Build history of the part. All positions in model axes, mm. Face numbers are marked on the shaded views. A direction names the side the tool comes from. Coordinates: 2 decimals unless noted, no trailing zeros. Loops run counter-clockwise (first coordinate to the right, second up) from the corner with the lowest first, then second, coordinate; pieces in that order, holes last.
Item 1: 3-axis set-ups, long thin cutter, end or side, ignore diameter. For the marked faces 1 and 2: which of +Z, -Z, +X, -X, +Y, -Y reach the whole face in a straight line?
Item 2: Cut at B-B (x = 44.5). List the corners of the cut face in (y, z) (1 decimal).
Item 3: Cut at A-A (x = -2.5). List the corners of the cut face in (y, z), and give its area (3 significant figures).
Item 4: Flat gauge pins, fed straight in: pin 1 (12 mm diameter, centred on x = 22.5, y = 11.5, fed in from -Z); pin 2 (2 mm diameter, centred on x = 75, z = -10, fed in from -Y); pin 3 (5 mm diameter, centred on y = 11, z = -5.5, fed in from +X). Where does each tip first touch, or does it go through?
Item 5: Drill centre lines: line 1 along X through (y, z) = (11.5, -8); line 2 along Z through (x, y) = (53, 0); line 3 along Y through (x, z) = (8, 3.5). Where is each one in solid material? Low to high.
Autodesk Inventor part; units mm, degrees
ref_plane "Work Plane1" through (1.525, 0, 0) normal (0, 0, 1) x (1, 0, 0)
ref_plane "YZ Plane" through (0, 0, 0) normal (1, 0, 0) x (0, 1, 0)
ref_plane "XZ Plane" through (0, 0, 0) normal (0, 1, 0) x (-1, 0, 0)
sketch "Sketch1" plane through (0, 0, 0) normal (0, 0, 1) x (1, 0, 0)
  line L0 (0, 16.4306) -> (0, 11.1125)
  line L1 (63.5, 11.1125) -> (101.6, 11.1125)
  line L2 (101.6, 11.1125) -> (101.6, 0)
  line L3 (101.6, 0) -> (-0.6351, 0)
  line L4 (-21.0821, 0) -> (122.047, 0)
  line L5 (-0.6351, 0) -> (-0.6351, 16.4306)
  line L6 (-0.6351, 16.4306) -> (0, 16.4306)
  line L7 (63.5, 11.1125) -> (61.7685, 11.1125)
  line L8 (61.7685, 11.1125) -> (0, 11.1125)
  line L9 (0, -3.2861) -> (0, 19.7168)
  dimension "d0" = 101.6
  dimension "d1" = 38.1
  dimension "d2" = 22.225
  dimension "d9" = 0.6351
  dimension "d10" = 32.8612
  dimension "d13" = 1.7315
  dimension "d14" = 22.225
revolve "Body" add sketch "Sketch1" angle 360 about axis through (101.6, 0, 0) along (-1, 0, 0)
sketch "Sketch2" plane through (-0.6351, 0, 0) normal (-1, 0, 0) x (0, 0, 1)
  line L0 (0, 21.0805) -> (18.2562, 10.5403)
  line L1 (18.2562, 10.5403) -> (18.2562, -10.5403)
  line L2 (18.2562, -10.5403) -> (0, -21.0805)
  line L3 (0, -21.0805) -> (-18.2562, -10.5403)
  line L4 (-18.2562, -10.5403) -> (-18.2562, 10.5403)
  line L5 (-18.2562, 10.5403) -> (0, 21.0805)
  point P0 (0, 0)
  point P1 (0, 0)
  dimension "d11" = 36.5125
extrude "Head" add sketch "Sketch2" along normal blind 13.2556
sketch "Sketch4" plane through (0, 0, 0) normal (0, 0, 1) x (1, 0, 0)
  line L0 (-13.8907, 18.2563) -> (-13.8907, 21.0805)
  line L1 (-13.8907, 21.0805) -> (-12.2601, 21.0805)
  line L2 (-12.2601, 21.0805) -> (-13.8907, 18.2563)
  line L3 (-16.5419, 0) -> (2.016, 0)
  line L4 (-0.6351, 21.0805) -> (-13.8907, 21.0805)
  line L5 (-13.8907, 10.5403) -> (-13.8907, 21.0805)
  dimension "d5" = 30
  dimension "d19" = 36.5125
revolve "Chamfer1" cut sketch "Sketch4" angle 360 about axis through (-10, 0, 0) along (1, 0, 0)
thread "Thread"
chamfer "Chamfer2" distance 1.7314 distance2 1.7315 1 edges at (101.6, -11.1125, 0) measured on face at (101.6, -3.0893, -3.2913)
ref_plane "Work Plane1" through (1.525, 0, 0) normal (0, 0, 1) x (1, 0, 0)
fillet "Fillet2" radius 1.5748 1 edges at (0, -11.1125, 0)
equation "\"d0\" = NLG"
equation "\"d1\" = GEL"
equation "\"d2\" = GD"
equation "\"d10\" = SD2"
equation "\"d14\" = BDM"
equation "\"d11\" = SW"
equation "\"d3\" = KOH - SD"
equation "\"d5\" = ANG1"
equation "\"d19\" = SW0"
equation "\"d63\" = R"
equation "\"d15\" = GEL"
equation "\"d6\" = -0.5 * SPD + 0.5 * GD"
equation "\"NLG\" = 101.6"
equation "\"GD\" = NND"
equation "\"BDM\" = 22.225"
equation "\"KOH\" = 13.89062"
equation "\"GEL\" = 38.1"
equation "\"SW\" = 36.5125"
equation "\"SW0\" = SW"
equation "\"SPD\" = GD1"
equation "\"SD2\" = 0.9 * SW"
equation "\"SD\" = 0.635"
equation "\"ANG1\" = 30deg"
equation "\"GAL\" = GUL"
equation "\"GUL\" = 1.73139"
equation "\"R\" = 1.5748"
equation "\"d62\" = -NLG - SD + GUL"
equation "\"GD1\" = 18.76222"
equation "\"THREADDIA\" = 22.225"
equation "\"TOA\" = 30deg"
equation "\"NND\" = 22.225"
equation "\"E0\" = 1.155 * SW"
properties part number "ANSI B18.2.6 - 7/8-9 UNC - 4" material "Steel, Mild"
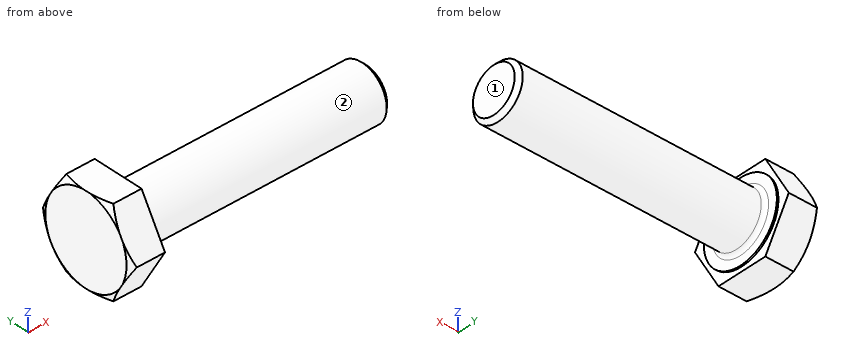
Filled sheet:
1. face 1: +Z, -Z, +X, +Y, -Y
1. face 2: +X
2. outline: circle Ø22.2 at (0, 0)
3. outline: (-21.08, 0) - (-10.54, -18.26) - (10.54, -18.26) - (21.08, 0) - (10.54, 18.26) - (-10.54, 18.26) - close
3. area: 1,150 mm2
4. pin 1: stops at z = -9.66
4. pin 2: stops at y = -6.52
4. pin 3: stops at x = 101.18
5. line 1: x = -13.89 to 0
5. line 2: z = -11.11 to 11.11
5. line 3: y = -10.55 to 10.55
